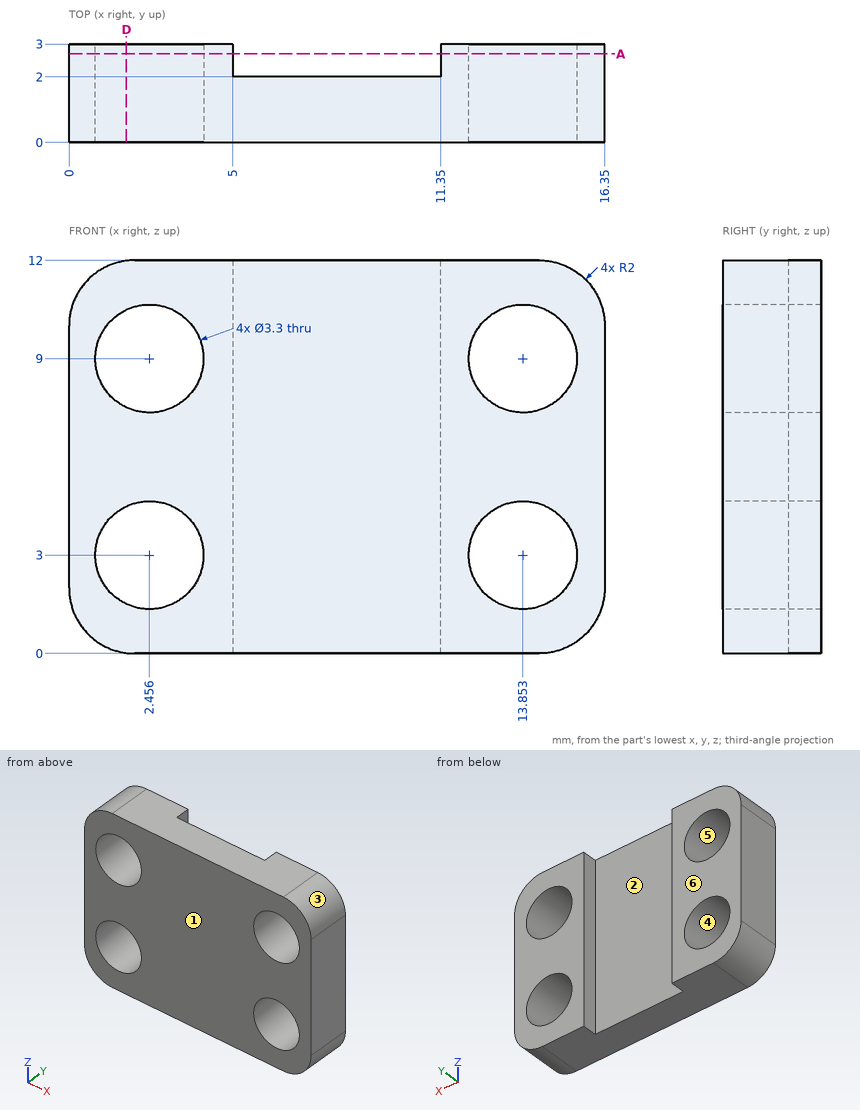
Could you check a few things on this drawing? It's one solid part, dimensions in mm from its lowest x, y, z. A direction names the side the tool comes from. Round coordinates to 2 decimals unless told otherwise and drop trailing zeros. Write each loop counter-clockwise with the first axis right and the second up, starting at its lowest first coordinate (ties: lowest second). Pieces come first, ordered by that corner, then holes. Notation, with made-up numbers: (-30.75, 5) -> (24.25, 5) arc R15 cw to (24.25, 15) -> close; hole circle Ø6 at (58, 62.5). An arc over 180 degrees is marked (long way). One line per question, with ' | ' between items. Start each with the question number.
1) I need wall thicknesses on line 1 (Z direction, x = 1, y = 0.8) (1 decimal); line 2 (X direction, y = 0.85, z = 10.25) (1 decimal); line 3 (Y direction, x = 6, z = 3). Which ranges of each line are inside material? Lowest first, please. Write a range as [from, to].
2) Suppose I cut it at D-D on x = 1.75. Write out the boundary of the cut face in (y, z) (1 decimal), then the cut area to 3 significant figures.
3) I'm going to push a flat-ended pin straight in: P1, Ø5, axis at x = 8, z = 3.5, coming from the +Y side. Where does the tip first touch, or does it pass through?
4) On a 3-axis mill with a long thin cutter (end or side, diameter ignored), from which of +Z, -Z, +X, -X, +Y, -Y can I reach the whole of each face in a straight line? I mean the marked faces 1 and 2. Say none if no direction works.
5) If we mould it in two halves opening along Z, with no side actions, what happens to the marked faces 3, 4, 5 and 6? For each: released by +Z, released by -Z, zero draft, split by the parting line, or undercut.
6) Suppose I cut it at A-A on y = 2.7. Count the separate pieces of the cut face and the enclosed holes in it.
Return value:
1) line 1: z = [0.3, 2.2], [3.8, 8.2], [9.8, 11.7] | line 2: x = [0, 1.4], [3.5, 12.8], [14.9, 16.3] | line 3: y = [0, 2]
2) outline: (0, 0) -> (3, 0) -> (3, 1.5) -> (0, 1.5) -> close; (0, 4.5) -> (3, 4.5) -> (3, 7.5) -> (0, 7.5) -> close; (0, 10.5) -> (3, 10.5) -> (3, 12) -> (0, 12) -> close | area: 18.0 mm2
3) P1: stops at y = 2
4) face 1: +Z, -Z, +X, -X, -Y | face 2: +Z, -Z, +Y
5) face 3: released by +Z | face 4: undercut | face 5: undercut | face 6: zero draft
6) separate pieces: 2 | enclosed holes: 4
